from build123d import *

# Parameters (mm, degrees)
BOSS_EXTRUDE1_DEPTH      = 25
BOSS_EXTRUDE1_DEPTH_BACK = 25
CUT_EXTRUDE1_DEPTH       = 17
CUT_EXTRUDE1_DEPTH_BACK  = 17
CUT_EXTRUDE2_DEPTH       = 8
CUT_EXTRUDE3_DEPTH       = 8
CUT_EXTRUDE4_DEPTH       = 21.5
CUT_EXTRUDE4_DEPTH_BACK  = 21.5
CUT_EXTRUDE5_DEPTH       = 35
CUT_EXTRUDE5_DEPTH_BACK  = 35
SKETCH7_W                = 107.768014059
SKETCH7_H                = 69.938488576
CUT_EXTRUDE6_DEPTH       = 29
CUT_EXTRUDE6_DEPTH_BACK  = 29


with BuildPart() as part:
    # Sketch1 → Boss-Extrude1 (new body, two sides)
    with BuildSketch(Plane.XY) as boss_extrude1_sk:
        with BuildLine():
            Line((-34.5, 0.2), (-31.366025404, 0.2))
            Line((-31.366025404, 0.2), (-30.5, 0.7))
            Line((-30.5, 0.7), (-21, 0.7))
            Line((-21, 0.7), (-21, 0))
            Line((-21, 0), (21, 0))
            Line((21, 0), (21, 0.7))
            Line((21, 0.7), (30.5, 0.7))
            Line((30.5, 0.7), (31.366025404, 0.2))
            Line((31.366025404, 0.2), (34.5, 0.2))
            ThreePointArc((34.5, 0.2), (34.853553391, 0.346446609), (35, 0.7))
            Line((35, 0.7), (34.913292535, 3.182976936))
            ThreePointArc((34.913292535, 3.182976936), (28.216815843, 6.59637195), (21, 8.696761129))
            Line((21, 8.696761129), (21, 11.9))
            Line((21, 11.9), (-21, 11.9))
            Line((-21, 11.9), (-21, 8.696761129))
            ThreePointArc((-21, 8.696761129), (-28.216815843, 6.59637195), (-34.913292535, 3.182976936))
            Line((-34.913292535, 3.182976936), (-35, 0.7))
            ThreePointArc((-35, 0.7), (-34.853553391, 0.346446609), (-34.5, 0.2))
        make_face()
    extrude(amount=BOSS_EXTRUDE1_DEPTH)
    extrude(boss_extrude1_sk.sketch, amount=-BOSS_EXTRUDE1_DEPTH_BACK)

    # Sketch2 → Cut-Extrude1 (cut, two sides)
    with BuildSketch(Plane.XY) as cut_extrude1_sk:
        with BuildLine():
            Line((21, 8.594559394), (21, 30))
            Line((21, 30), (-21, 30))
            Line((-21, 30), (-21, 8.594559394))
            ThreePointArc((-21, 8.594559394), (0, 11.4), (21, 8.594559394))
        make_face()
    extrude(amount=CUT_EXTRUDE1_DEPTH, mode=Mode.SUBTRACT)
    extrude(cut_extrude1_sk.sketch, amount=-CUT_EXTRUDE1_DEPTH_BACK, mode=Mode.SUBTRACT)

    # Sketch3 → Cut-Extrude2 (cut)
    with BuildSketch(Plane.XY.offset(25)):
        Polygon((-21.5, -3), (-21, -3), (-21, 6.37), (-19.5, 7.87), (-19.5, 8.9), (-21, 8.9), (-21, 11.9), (21, 11.9), (21, 8.9), (19.5, 8.9), (19.5, 7.87), (21, 6.37), (21, -3), (21.5, -3), (21.5, 16.9), (-21.5, 16.9), align=None)
    extrude(amount=-CUT_EXTRUDE2_DEPTH, mode=Mode.SUBTRACT)

    # Sketch4 → Cut-Extrude3 (cut)
    with BuildSketch(Plane.XY.offset(-25)):
        Polygon((-21.5, -3), (-21, -3), (-21, 6.37), (-19.5, 7.87), (-19.5, 8.9), (-21, 8.9), (-21, 11.9), (21, 11.9), (21, 8.9), (19.5, 8.9), (19.5, 7.87), (21, 6.37), (21, -3), (21.5, -3), (21.5, 16.9), (-21.5, 16.9), align=None)
    extrude(amount=CUT_EXTRUDE3_DEPTH, mode=Mode.SUBTRACT)

    # Sketch5 → Cut-Extrude4 (cut, two sides)
    with BuildSketch(Plane(origin=(0, 0, 0), x_dir=(0, 0, -1), z_dir=(1, 0, 0))) as cut_extrude4_sk:
        Polygon((-17, 8.25), (-16.5, 8.25), (-16.5, 11), (16.5, 11), (16.5, 8.25), (17, 8.25), (17, 12), (-17, 12), align=None)
    extrude(amount=CUT_EXTRUDE4_DEPTH, mode=Mode.SUBTRACT)
    extrude(cut_extrude4_sk.sketch, amount=-CUT_EXTRUDE4_DEPTH_BACK, mode=Mode.SUBTRACT)

    # Sketch6 → Cut-Extrude5 (cut, two sides)
    with BuildSketch(Plane(origin=(0, 0, 0), x_dir=(0, 0, -1), z_dir=(1, 0, 0))) as cut_extrude5_sk:
        with BuildLine():
            Line((-30, 1.2), (-30, -5))
            Line((-30, -5), (30, -5))
            Line((30, -5), (30, 1.2))
            Line((30, 1.2), (14.5, 1.2))
            ThreePointArc((14.5, 1.2), (13.792893219, 0.907106781), (13.5, 0.2))
            Line((13.5, 0.2), (13.5, -2))
            Line((13.5, -2), (-13.5, -2))
            Line((-13.5, -2), (-13.5, 0.2))
            ThreePointArc((-13.5, 0.2), (-13.792893219, 0.907106781), (-14.5, 1.2))
            Line((-14.5, 1.2), (-30, 1.2))
        make_face()
    extrude(amount=CUT_EXTRUDE5_DEPTH, mode=Mode.SUBTRACT)
    extrude(cut_extrude5_sk.sketch, amount=-CUT_EXTRUDE5_DEPTH_BACK, mode=Mode.SUBTRACT)

    # Sketch7 → Cut-Extrude6 (cut, two sides)
    with BuildSketch(Plane(origin=(0, 0, 0), x_dir=(-1, 0, 0), z_dir=(0, 1, 0))) as cut_extrude6_sk:
        with Locations((-2.122144112, 2.214411248)):
            Rectangle(SKETCH7_W, SKETCH7_H)
        with BuildLine():
            Line((35, -20), (35, 20))
            ThreePointArc((35, 20), (33.535533906, 23.535533906), (30, 25))
            Line((30, 25), (-30, 25))
            ThreePointArc((-30, 25), (-33.535533906, 23.535533906), (-35, 20))
            Line((-35, 20), (-35, -20))
            ThreePointArc((-35, -20), (-33.535533906, -23.535533906), (-30, -25))
            Line((-30, -25), (30, -25))
            ThreePointArc((30, -25), (33.535533906, -23.535533906), (35, -20))
        make_face(mode=Mode.SUBTRACT)
    extrude(amount=CUT_EXTRUDE6_DEPTH, mode=Mode.SUBTRACT)
    extrude(cut_extrude6_sk.sketch, amount=-CUT_EXTRUDE6_DEPTH_BACK, mode=Mode.SUBTRACT)

    # Sketch8 → Cut-Revolve1 (revolve, cut)
    with BuildSketch(Plane.XY.offset(21)):
        Polygon((-17, 2.364115214), (-18.621, 3.3), (-18.621, 11.521), (-19, 11.9), (-17, 11.9), align=None)
    revolve(axis=Axis((-17, 11.9, 21), (0, -1, 0)), mode=Mode.SUBTRACT)

    # Sketch9 → Cut-Revolve2 (revolve, cut)
    with BuildSketch(Plane.XY.offset(-21)):
        Polygon((-17, 2.364115214), (-18.621, 3.3), (-18.621, 11.521), (-19, 11.9), (-17, 11.9), align=None)
    revolve(axis=Axis((-17, 11.9, -21), (0, -1, 0)), mode=Mode.SUBTRACT)

    # Sketch10 → Cut-Revolve3 (revolve, cut)
    with BuildSketch(Plane.XY.offset(-21)):
        Polygon((17, 2.364115214), (15.379, 3.3), (15.379, 11.521), (15, 11.9), (17, 11.9), align=None)
    revolve(axis=Axis((17, 11.9, -21), (0, -1, 0)), mode=Mode.SUBTRACT)

    # Sketch11 → Cut-Revolve4 (revolve, cut)
    with BuildSketch(Plane.XY.offset(21)):
        Polygon((17, 2.364115214), (15.379, 3.3), (15.379, 11.521), (15, 11.9), (17, 11.9), align=None)
    revolve(axis=Axis((17, 11.9, 21), (0, -1, 0)), mode=Mode.SUBTRACT)

    # Sketch12 → Cut-Revolve5 (revolve, cut)
    with BuildSketch(Plane.XY.offset(21)):
        Polygon((0, 4.745299462), (-2, 5.9), (-2, 11.9), (0, 11.9), align=None)
    revolve(axis=Axis((0, 11.9, 21), (0, -1, 0)), mode=Mode.SUBTRACT)

    # Sketch13 → Cut-Revolve6 (revolve, cut)
    with BuildSketch(Plane.XY.offset(-21)):
        Polygon((0, 4.745299462), (-2, 5.9), (-2, 11.9), (0, 11.9), align=None)
    revolve(axis=Axis((0, 11.9, -21), (0, -1, 0)), mode=Mode.SUBTRACT)


solid = part.part
Model file for the job. Use its own axes, mm. A direction names the side the tool comes from. Give positions to 0.01 mm unless a question says otherwise; leave off trailing zeros. Loops run counter-clockwise (first coordinate to the right, second up) from the corner with the lowest first, then second, coordinate; pieces in that order, holes last.
1) Tool access for faces 1 (the flat face through (-21, 4, -21)), 2 (the flat face through (20, 8.9, 21)), 3 (the flat face through (-21.2, 5.5, -17)), 4 (the cylindrical face through (0, 9, -23)): list every direction of +Z, -Z, +X, -X, +Y, -Y with a clear straight run to the whole face (end or side of a thin tool).
2) Wall check: line 1 (Z direction, x = 0, y = 8.4); line 2 (Z direction, x = 0, y = 7.75); line 3 (X direction, y = 9.3, z = 21). Give the ranges that are in metal, low to high.
3) Pull direction Z, two halves, no side cores. Call faces 5 (the flat face through (-26, 4, 25)), 6 (the cylindrical face through (15.503, 7.468, -20.379)), 7 (the flat face through (20, 8.9, -21)): +Z half, -Z half, draft (parallel to the pull), parting line (faces both ways), or undercut.
4) Flat gauge pins, fed straight in: pin 1 Ø1.6 at (y, z) = (5, 20) entering from -X; pin 2 Ø3.5 at (y, z) = (11, 21) entering from -X; pin 3 Ø3 at (x, z) = (15, 8.5) entering from +Y; pin 4 Ø1 at (x, z) = (-5.5, 4.5) entering from -Y. Where does each tip first touch, or does it go through?
5) Saw through at C-C (x = -28.5). Write the cut outline in (y, z), plus the area to 3 significant figures.
6) Saw through at A-A (y = 10). Count the separate pieces of the cut face and the enclosed holes in it, plus the area to 3 significant figures.
7) Saw through at B-B (z = -12.5). Write the cut outline in (x, y), plus the area to 3 significant figures.
Answer block:
1. face 1: -Z, +Y, -Y
1. face 2: +Z, +X
1. face 3: -Z
1. face 4: +Y
2. line 1: z = -25 to -23, -19 to -17, -16.5 to 16.5, 17 to 19, 23 to 25
2. line 2: z = -25 to -23, -19 to 19, 23 to 25
2. line 3: x = -21 to -18.62, -15.38 to -2, 2 to 15.38, 18.62 to 21
3. face 5: +Z half
3. face 6: undercut
3. face 7: draft
4. pin 1: stops at x = -33.22
4. pin 2: stops at x = -21
4. pin 3: stops at y = 10.25
4. pin 4: stops at y = 0
5. outline: (0.7, -13.63) arc R1 cw to (1.2, -14.5) - (1.2, -25) - (6.48, -25) - (6.48, 25) - (1.2, 25) - (1.2, 14.5) arc R1 cw to (0.7, 13.63) - close
5. area: 278 mm2
6. separate pieces: 3
6. enclosed holes: 6
6. area: 1,600 mm2
7. outline: (-35, 0.7) arc R0.5 ccw to (-34.5, 0.2) - (-31.37, 0.2) - (-30.5, 0.7) - (-21, 0.7) - (-21, 0) - (21, 0) - (21, 0.7) - (30.5, 0.7) - (31.37, 0.2) - (34.5, 0.2) arc R0.5 ccw to (35, 0.7) - (34.91, 3.18) arc R40 ccw to (21, 8.7) - (21, 8.59) arc R80 ccw to (7.99, 11) - (-7.99, 11) arc R80 ccw to (-21, 8.59) - (-21, 8.7) arc R40 ccw to (-34.91, 3.18) - close
7. area: 600 mm2
